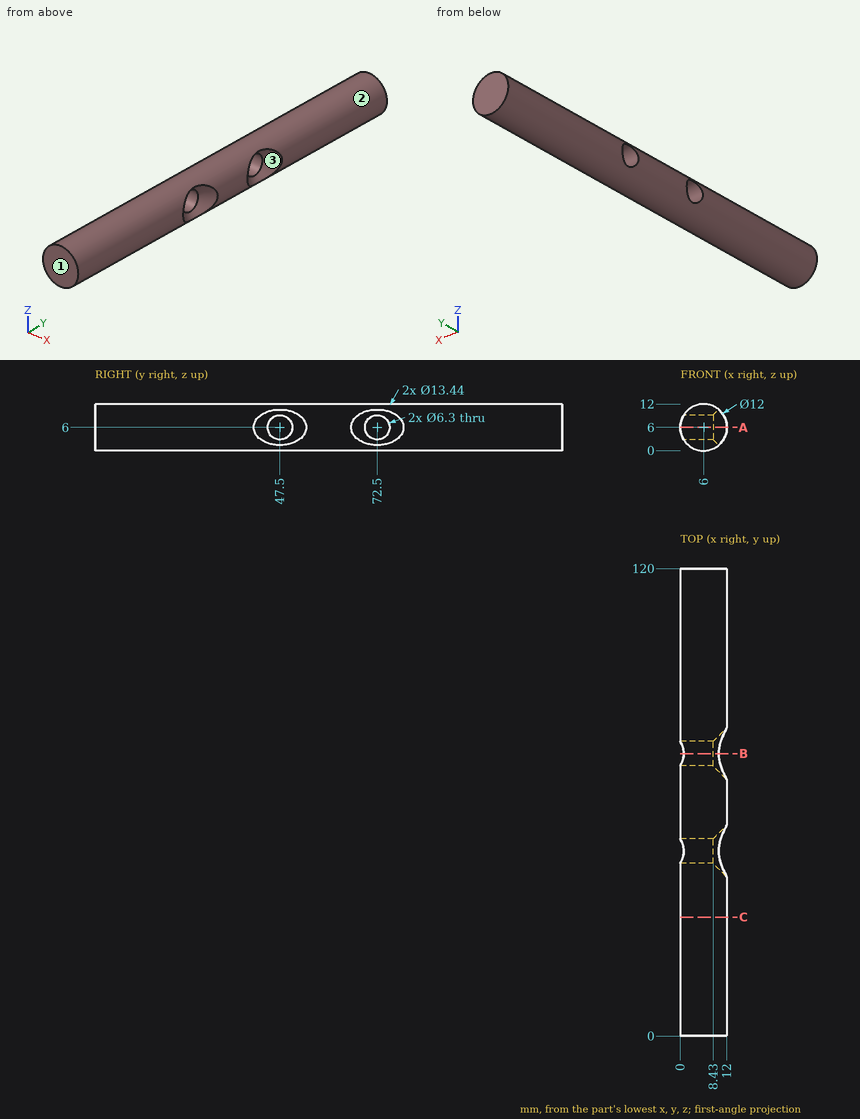
The drawing under review shows one solid part. Ordinate dimensions are in mm from its lowest x, y, z. Coordinates: 2 decimals unless noted, no trailing zeros. Order: outer loops, then holes, each group sorted by start corner. A loop starts at its lowest first (then second) coordinate and runs counter-clockwise, first axis right, second up. Notation, with made-up numbers: M 62,62 L 67,62 A19 ccw 67,80 Z; hole C -9,-22 d10. An arc over 180 degrees is marked long. One line per question, with ' | ' between items.
(1) Add section C-C, the plane y = 30.5. Write out the cut boundary in (x, z).
Geometry results:
outline: C 6,6 d12
(2) Add section B-B, the plane y = 72.5. Write out the cut boundary in (x, z), then the cut area to 3 significant figures.
Geometry results:
outline: M 0.89,2.85 A6 ccw 9.87,1.41 L 8.43,2.85 Z; M 0.89,9.15 L 8.43,9.15 L 9.87,10.59 A6 ccw Z | area: 37.1 mm²
(3) Add section A-A, the plane z = 6. Write out the cut boundary in (x, y).
Geometry results:
outline: M 0,0 L 12,0 L 12,40.78 L 8.43,44.35 L 0,44.35 Z; M 0,50.65 L 8.43,50.65 L 12,54.22 L 12,65.78 L 8.43,69.35 L 0,69.35 Z; M 0,75.65 L 8.43,75.65 L 12,79.22 L 12,120 L 0,120 Z
(4) For probe 1 along Z at (x, y) = (6.5, 106.5); probe 2 along Z at (x, y) = (4.25, 72.5); probe 3 along Y at (x, z) = (7.25, 6.75), list the stretches that pass through material, from the lowest coordinate up. Write a range as from..to.
Geometry results:
probe 1: z = 0.02..11.98 | probe 2: z = 0.26..2.85, 9.15..11.74 | probe 3: y = 0..44.44, 50.56..69.44, 75.56..120
(5) Insertion check: pin 1 (2 mm diameter, centred on x = 4.5, y = 17.5, fed in from +Z); pin 2 (3 mm diameter, centred on y = 75, z = 9.5, fed in from +X). Each pin has a flat end and moves straight along its axis. Give the tip position at first contact, or say it passes through.
Geometry results:
pin 1: stops at z = 11.98 | pin 2: stops at x = 10.72
(6) The part is to be moulded in two halves that separate along Z. For the marked faces 1, 2 and 3, say which applies: +Z half, -Z half, draft (parallel to the pull), parting line (faces both ways), or undercut.
Geometry results:
face 1: draft | face 2: parting line | face 3: undercut
